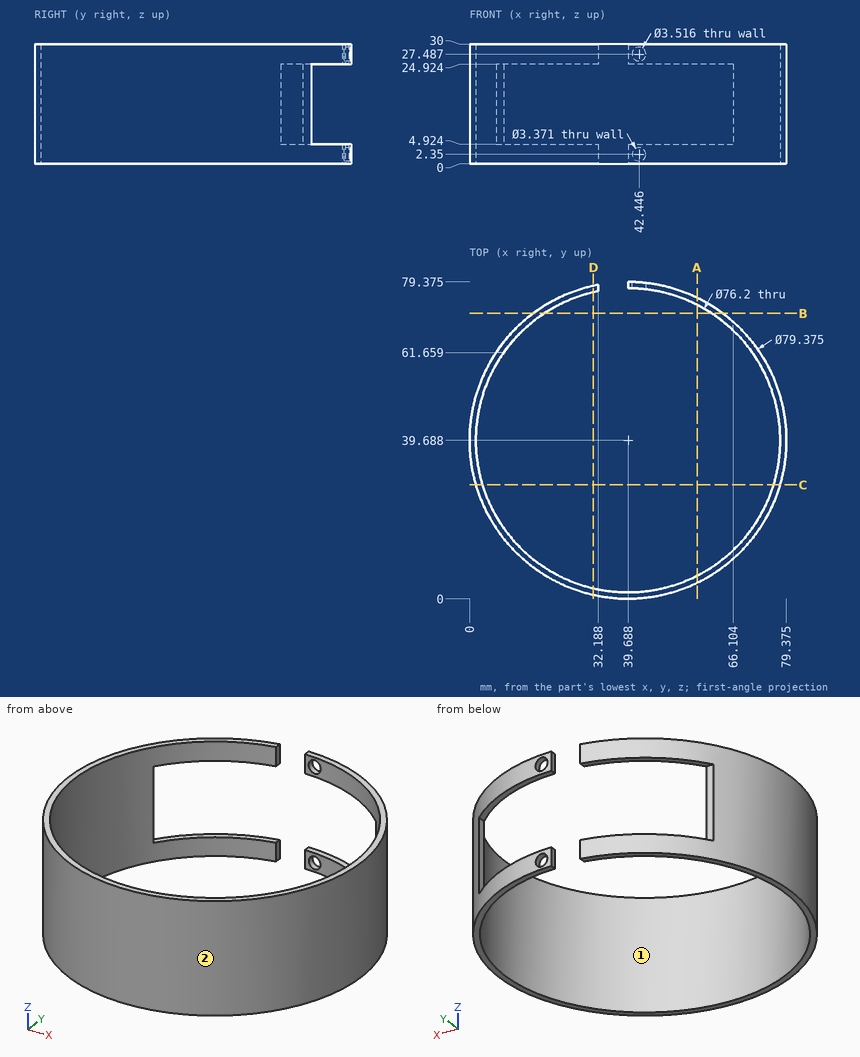
Here's the drawing with two shaded views (mm, measured from the low corner). I have some questions. Give positions to 0.01 mm unless a question says otherwise; leave off trailing zeros. Write each loop counter-clockwise with the first axis right and the second up, starting at its lowest first coordinate (ties: lowest second). Pieces come first, ordered by that corner, then holes. Notation, with made-up numbers: (-39, -6) -> (-33, -6) arc R20 cw to (-33, 18) -> close; hole circle Ø4 at (33, 80.25). An arc over 180 degrees is marked (long way). Use one line per item in the form item = value. Start each with the question number.
1. If I drill on L1, parallel to Z at x = 19, y = 73 (1 decimal); L2, parallel to X at y = 37, z = 14 (1 decimal); L3, parallel to Y at x = 6, z = 25 (1 decimal), over which ranges is the centre line in solid material (lowest first)?
2. Imagine slicing it at C-C on y = 28.5. List the corners of the cut face in (x, z) for me (1 decimal).
3. Thinking about a two-plate mould opening in Y: for the marked faces 1 and 2, which applies, +Y half, -Y half, draft (parallel to the pull), parting line (faces both ways), or undercut?
4. Imagine slicing it at A-A on x = 57. List the corners of the cut face in (y, z) for me (1 decimal).
5. Will these pins go through, and if not, where does the flat tip stop? pin 1 Ø2 at (x, z) = (31.5, 3.5) entering from -Y; pin 2 Ø4 at (x, z) = (42.45, 27.49) entering from +Y; pin 3 Ø2 at (x, z) = (67, 8.5) entering from +Y.
6. Imagine slicing it at B-B on y = 71.5. List the corners of the cut face in (x, z) for me (1 decimal).
7. Imagine slicing it at D-D on x = 31. List the corners of the cut face in (y, z) for me (1 decimal).
Entries:
q1.L1 = 0 to 4.9, 24.9 to 30
q1.L2 = 0.1 to 1.7, 77.7 to 79.3
q1.L3 = 18.7 to 21.9, 57.5 to 60.7
q2.outline = (1.6, 0) -> (3.3, 0) -> (3.3, 30) -> (1.6, 30) -> close; (76.1, 0) -> (77.8, 0) -> (77.8, 30) -> (76.1, 30) -> close
q3.face_1 = undercut
q3.face_2 = parting line
q4.outline = (4, 0) -> (5.7, 0) -> (5.7, 30) -> (4, 30) -> close; (73.6, 0) -> (75.4, 0) -> (75.4, 4.9) -> (73.6, 4.9) -> close; (73.6, 24.9) -> (75.4, 24.9) -> (75.4, 30) -> (73.6, 30) -> close
q5.pin_1 = 0.66
q5.pin_2 = 79.37
q5.pin_3 = 69.31
q6.outline = (16, 0) -> (18.7, 0) -> (18.7, 4.9) -> (16, 4.9) -> close; (16, 24.9) -> (18.7, 24.9) -> (18.7, 30) -> (16, 30) -> close; (60.7, 0) -> (63.4, 0) -> (63.4, 4.9) -> (60.7, 4.9) -> close; (60.7, 24.9) -> (63.4, 24.9) -> (63.4, 30) -> (60.7, 30) -> close
q7.outline = (1, 0) -> (2.6, 0) -> (2.6, 30) -> (1, 30) -> close; (76.8, 0) -> (78.4, 0) -> (78.4, 4.9) -> (76.8, 4.9) -> close; (76.8, 24.9) -> (78.4, 24.9) -> (78.4, 30) -> (76.8, 30) -> close
